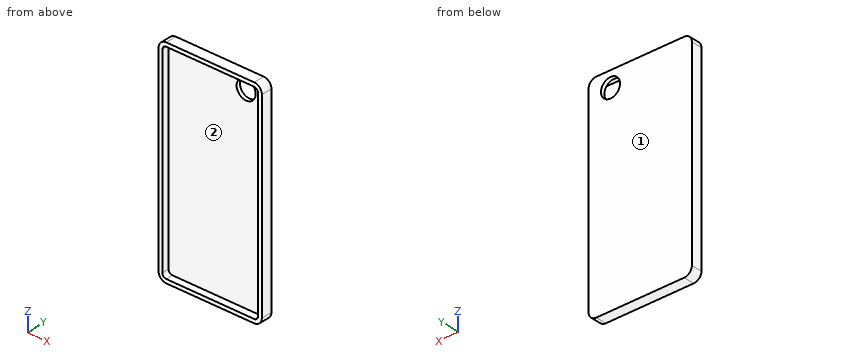
from build123d import *

# Parameters (mm, degrees)
F0_W     = 67.1
F0_H     = 138.3
F1_DEPTH = 3.55
F2_R     = 5
F3_T     = -2.5
F4_R     = 6.1900061573
F5_DEPTH = 12.5


with BuildPart() as f1:
    # F0 (on Front) → F1 (new body, symmetric)
    with BuildSketch(Plane.XZ):
        Rectangle(F0_W, F0_H)
    extrude(amount=F1_DEPTH, both=True)

    # F2
    f2_edges = [f1.edges().sort_by_distance(p)[0] for p in [
        (-33.55, 0, 69.15),
        (33.55, 0, 69.15),
        (33.55, 0, -69.15),
        (-33.55, 0, -69.15),
    ]]
    fillet(f2_edges, radius=F2_R)

    # F3
    f3_openings = [f1.faces().sort_by_distance(p)[0] for p in [
        (0, -3.55, 0),
    ]]
    offset(amount=F3_T, openings=f3_openings)

    # F4 (on Front) → F5 (cut, symmetric)
    with BuildSketch(Plane.XZ):
        with Locations((19.3064566702, 59.0549409389)):
            Circle(F4_R)
    extrude(amount=F5_DEPTH, both=True, mode=Mode.SUBTRACT)


solid = f1.part
Build history of the part. All positions in model axes, mm. Face numbers are marked on the shaded views. Round coordinates to 2 decimals unless told otherwise and drop trailing zeros. Loops run counter-clockwise (first coordinate to the right, second up) from the corner with the lowest first, then second, coordinate; pieces in that order, holes last. Notation, with made-up numbers: (1.25, -25) -> (9.25, -25) arc R14 cw to (9.25, 1) -> close; hole circle Ø8 at (-13, 25.25). An arc over 180 degrees is marked (long way). Use CSV: the item, a comma, the result in double quotes. Start each with the question number.
Q1. Saw through at A-A on y = -0.5. Give the cut face in (x, z).
Q2. Mould opens along X. For the marked faces 1 and 2 say: +X half, -X half, draft (parallel to the pull), parting line (faces both ways), or undercut.
Q3. Drill centre lines: L1, parallel to X at y = 0.25, z = -19; L2, parallel to Z at x = 9.5, y = 0.5; L3, parallel to Y at x = -4.5, z = 35.5. Where is each one in solid material? Low to high.
Q4. Saw through at D-D on z = -5.5. Give the cut face in (x, y).
Q5. Saw through at C-C on x = 17.5. Give the cut face in (y, z).
Q6. Flat gauge pin, fed straight in: pin 1 Ø2 at (x, z) = (3, 26) entering from -Y. Where does the tip first touch, or does it go through?
Q7. Saw through at B-B on z = 56.5. Give the cut face in (x, y).
Solutions:
1,outline,"(-33.55, -64.15) arc R5 ccw to (-28.55, -69.15) -> (28.55, -69.15) arc R5 ccw to (33.55, -64.15) -> (33.55, 64.15) arc R5 ccw to (28.55, 69.15) -> (-28.55, 69.15) arc R5 ccw to (-33.55, 64.15) -> close; hole (-31.05, -64.15) arc R2.5 ccw to (-28.55, -66.65) -> (28.55, -66.65) arc R2.5 ccw to (31.05, -64.15) -> (31.05, 64.15) arc R2.5 ccw to (28.55, 66.65) -> (-28.55, 66.65) arc R2.5 ccw to (-31.05, 64.15) -> close"
2,face 1,"draft"
2,face 2,"undercut"
3,L1,"x = -33.55 to -31.05, 31.05 to 33.55"
3,L2,"z = -69.15 to -66.65, 66.65 to 69.15"
3,L3,"y = 1.05 to 3.55"
4,outline,"(-33.55, -3.55) -> (-31.05, -3.55) -> (-31.05, 1.05) -> (31.05, 1.05) -> (31.05, -3.55) -> (33.55, -3.55) -> (33.55, 3.55) -> (-33.55, 3.55) -> close"
5,outline,"(-3.55, -69.15) -> (3.55, -69.15) -> (3.55, 53.13) -> (1.05, 53.13) -> (1.05, -66.65) -> (-3.55, -66.65) -> close; (-3.55, 66.65) -> (1.05, 66.65) -> (1.05, 64.98) -> (3.55, 64.98) -> (3.55, 69.15) -> (-3.55, 69.15) -> close"
6,pin 1,"stops at y = 1.05"
7,outline,"(-33.55, -3.55) -> (-31.05, -3.55) -> (-31.05, 1.05) -> (13.67, 1.05) -> (13.67, 3.55) -> (-33.55, 3.55) -> close; (24.94, 1.05) -> (31.05, 1.05) -> (31.05, -3.55) -> (33.55, -3.55) -> (33.55, 3.55) -> (24.94, 3.55) -> close"
